from build123d import *

# Parameters (mm, degrees)
SKETCH_1_R      = 1.6
SKETCH_1_R_2    = 1.1
EXTRUDE_1_DEPTH = 3
FILLET_1_R      = 2


with BuildPart() as part:
    # 草图1 → 凸台-拉伸1 (new body)
    with BuildSketch(Plane(origin=(0, 0, 0), x_dir=(1, 0, 0), z_dir=(0, 1, 0))):
        with BuildLine():
            Line((-36, 10), (-36, 0))
            Line((-36, 0), (36, 0))
            Line((36, 0), (36, 10))
            Line((36, 10), (16.121320344, 10))
            ThreePointArc((16.121320344, 10), (15.060660172, 9.560660172), (14, 10))
            ThreePointArc((14, 10), (13.560916248, 11.032944403), (13.961534907, 12.081406787))
            ThreePointArc((13.961534907, 12.081406787), (13.212832412, 19.384450727), (11.520782396, 26.528117359))
            ThreePointArc((11.520782396, 26.528117359), (8, 50), (11.520782396, 73.471882641))
            ThreePointArc((11.520782396, 73.471882641), (13.376747878, 81.643487818), (14, 90))
            Line((14, 90), (14, 97.5))
            Line((14, 97.5), (-14, 97.5))
            Line((-14, 97.5), (-14, 90))
            ThreePointArc((-14, 90), (-13.376747878, 81.643487818), (-11.520782396, 73.471882641))
            ThreePointArc((-11.520782396, 73.471882641), (-8, 50), (-11.520782396, 26.528117359))
            ThreePointArc((-11.520782396, 26.528117359), (-13.212832412, 19.384450727), (-13.961534907, 12.081406787))
            ThreePointArc((-13.961534907, 12.081406787), (-13.664471091, 11.608981293), (-13.560660172, 11.060660172))
            ThreePointArc((-13.560660172, 11.060660172), (-13.674840873, 10.486635023), (-14, 10))
            ThreePointArc((-14, 10), (-15.060660172, 9.560660172), (-16.121320344, 10))
            Line((-16.121320344, 10), (-36, 10))
        make_face()
        with Locations(Location((-28.5, 5, 0), (0, 0, 270))):
            Circle(SKETCH_1_R, mode=Mode.SUBTRACT)
        with Locations(Location((-6.5, 20.5, 0), (0, 0, 270))):
            Circle(SKETCH_1_R, mode=Mode.SUBTRACT)
        with Locations(Location((6.5, 20.5, 0), (0, 0, 270))):
            Circle(SKETCH_1_R, mode=Mode.SUBTRACT)
        with Locations(Location((28.5, 5, 0), (0, 0, 270))):
            Circle(SKETCH_1_R, mode=Mode.SUBTRACT)
        with Locations(Location((0, 25, 0), (0, 0, 270))):
            Circle(SKETCH_1_R_2, mode=Mode.SUBTRACT)
        with Locations(Location((0, 40, 0), (0, 0, 270))):
            Circle(SKETCH_1_R_2, mode=Mode.SUBTRACT)
        with Locations(Location((-10, 93.5, 0), (0, 0, 270))):
            Circle(SKETCH_1_R, mode=Mode.SUBTRACT)
        with Locations(Location((0, 55, 0), (0, 0, 270))):
            Circle(SKETCH_1_R_2, mode=Mode.SUBTRACT)
        with Locations(Location((0, 70, 0), (0, 0, 270))):
            Circle(SKETCH_1_R_2, mode=Mode.SUBTRACT)
        with Locations(Location((0, 85, 0), (0, 0, 270))):
            Circle(SKETCH_1_R_2, mode=Mode.SUBTRACT)
        with Locations(Location((10, 93.5, 0), (0, 0, 270))):
            Circle(SKETCH_1_R, mode=Mode.SUBTRACT)
    extrude(amount=EXTRUDE_1_DEPTH)

    # 圆角1
    fillet_1_edges = [part.edges().sort_by_distance(p)[0] for p in [
        (36, 1.5, -10),
        (36, 1.5, 0),
        (-36, 1.5, 0),
        (-36, 1.5, -10),
        (-14, 1.5, -97.5),
        (14, 1.5, -97.5),
    ]]
    fillet(fillet_1_edges, radius=FILLET_1_R)


solid = part.part
Source: CAD feature listing. Evaluate the final solid. Frame: model axes, mm. A direction names the side the tool comes from. Give positions to 0.01 mm unless a question says otherwise; leave off trailing zeros. Order: outer loops, then holes, each group sorted by start corner. A loop starts at its lowest first (then second) coordinate and runs counter-clockwise, first axis right, second up. Notation, with made-up numbers: (17.25, 26) -> (72.25, 26) arc R14 ccw to (72.25, 33) -> close; hole circle Ø8 at (-30.5, -8.5). An arc over 180 degrees is marked (long way). Write item = value, one per line.
Item 1: Set-up query: faces 1 (the face through (-25, 1, -10)), 2 (the face through (-13.4, 1.5, -81.8)), 3 (the face through (10.07, 1.48, -95.1)). Return all of +Z, -Z, +X, -X, +Y, -Y with unobstructed straight access to the full face (end or side cutting, diameter ignored); none if empty.
Check result:
face_1 = -Z, -X, +Y, -Y
face_2 = -X, +Y, -Y
face_3 = +Y, -Y
Item 2: Contact query for flat-ended pins moving along their axis: pin 1 (0.9 mm diameter, centred on y = 2, z = -92, fed in from +X); pin 2 (1.5 mm diameter, centred on x = 29, y = 2, fed in from -Z); pin 3 (1.5 mm diameter, centred on y = 2, z = -56.5, fed in from -X). Output: stop coordinate, or through.
Check result:
pin_1 = 14
pin_2 = -10
pin_3 = -8.33
Item 3: Section query C-C (z = -70). Output: boundary loops of the cut face in (x, y), then the cut area to 3 significant figures.
Check result:
outline = (-10.54, 0) -> (-1.1, 0) -> (-1.1, 3) -> (-10.54, 3) -> close; (1.1, 0) -> (10.54, 0) -> (10.54, 3) -> (1.1, 3) -> close
area = 56.6 mm²
Item 4: Section query A-A (x = -6.5). Output: boundary loops of the cut face in (y, z).
Check result:
outline = (0, -97.5) -> (3, -97.5) -> (3, -22.1) -> (0, -22.1) -> close; (0, -18.9) -> (3, -18.9) -> (3, 0) -> (0, 0) -> close
Item 5: Ray query, probe 1 along X at (y, z) = (1.65, -93.5); probe 2 along X at (y, z) = (1.1, -20.5); probe 3 along X at (y, z) = (1.2, -40). Return the intervals inside material, ascending.
Check result:
probe_1 = -14 to -11.6, -8.4 to 8.4, 11.6 to 14
probe_2 = -13.01 to -8.1, -4.9 to 4.9, 8.1 to 13.01
probe_3 = -8.63 to -1.1, 1.1 to 8.63
Item 6: Section query B-B (z = -93.5). Output: boundary loops of the cut face in (x, y), then the cut area to 3 significant figures.
Check result:
outline = (-14, 0) -> (-11.6, 0) -> (-11.6, 3) -> (-14, 3) -> close; (-8.4, 0) -> (8.4, 0) -> (8.4, 3) -> (-8.4, 3) -> close; (11.6, 0) -> (14, 0) -> (14, 3) -> (11.6, 3) -> close
area = 64.8 mm²
Item 7: Section query D-D (x = 25). Output: boundary loops of the cut face in (y, z).
Check result:
outline = (0, -10) -> (3, -10) -> (3, 0) -> (0, 0) -> close
Item 8: Mould query, pull axis Z, two halves, no side actions, for faces 4 (the face through (-35.43, 1.52, -0.6)), 5 (the face through (14, 1, -93)), 6 (the face through (25, 1, -10)), 7 (the face through (-8.06, 1.48, -20.85)). Classes: +Z half, -Z half, draft (parallel to the pull), parting line (faces both ways), or undercut.
Check result:
face_4 = +Z half
face_5 = draft
face_6 = -Z half
face_7 = undercut
